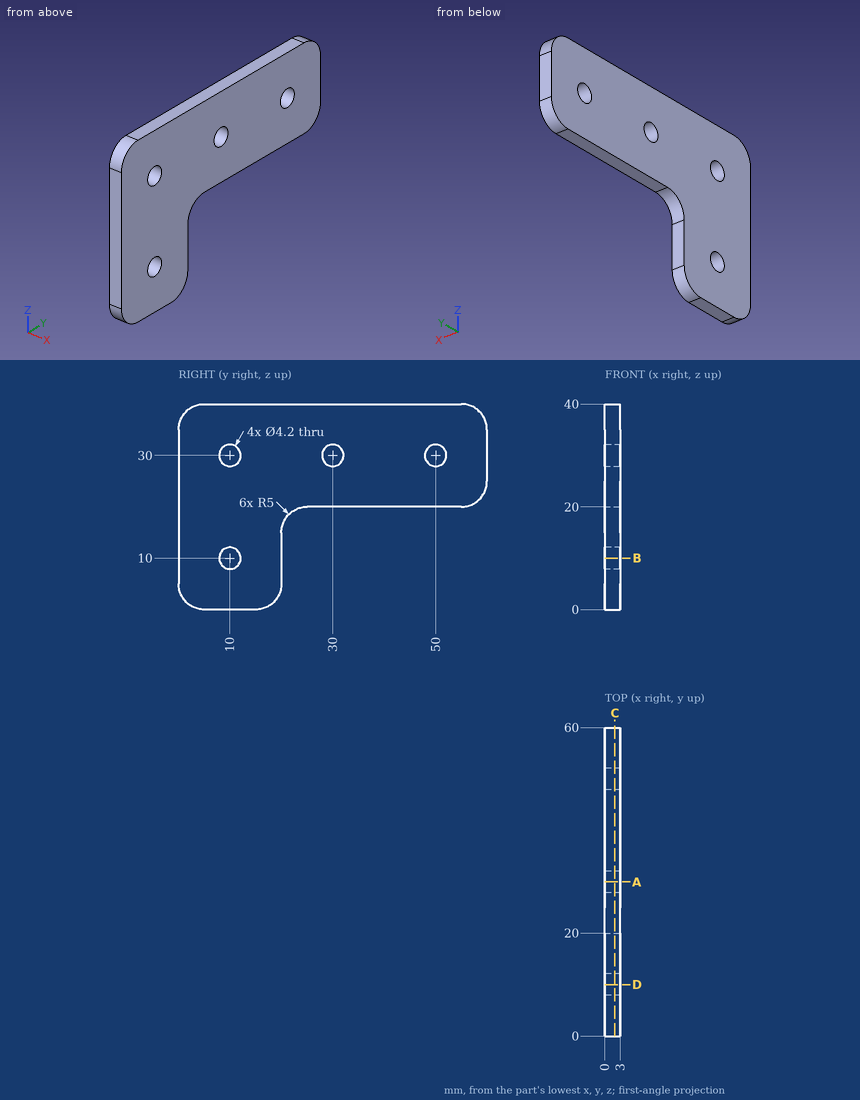
Source: three-view drawing plus pictorial views. Frame: mm from the lowest corner of the part. Give positions to 0.01 mm unless a question says otherwise; leave off trailing zeros. Order: outer loops, then holes, each group sorted by start corner. A loop starts at its lowest first (then second) coordinate and runs counter-clockwise, first axis right, second up. Notation, with made-up numbers: M 65.25,46.25 L 90.25,46.25 A26 ccw 90.25,73.25 Z; hole C 8.5,1 d4. An arc over 180 degrees is marked long. Return JSON: item names as keys, results as strings.
1) Section query D-D on y = 10. Output: boundary loops of the cut face in (x, z).
Taken from the geometry:
{"outline": "M 0,0 L 3,0 L 3,7.9 L 0,7.9 Z; M 0,12.1 L 3,12.1 L 3,27.9 L 0,27.9 Z; M 0,32.1 L 3,32.1 L 3,40 L 0,40 Z"}
2) Line query: L1, parallel to Y at x = 2.2, z = 30; L2, parallel to Z at x = 0.3, y = 54; L3, parallel to Z at x = 2.55, y = 11.5. Output: solid intervals per line, ascending. Write a range as [from, to].
Taken from the geometry:
{"L1": "y = [0, 7.9], [12.1, 27.9], [32.1, 47.9], [52.1, 60]", "L2": "z = [20, 40]", "L3": "z = [0, 8.53], [11.47, 28.53], [31.47, 40]"}
3) Section query B-B on z = 10. Output: boundary loops of the cut face in (x, y), and give its area (3 significant figures).
Taken from the geometry:
{"outline": "M 0,0 L 3,0 L 3,7.9 L 0,7.9 Z; M 0,12.1 L 3,12.1 L 3,20 L 0,20 Z", "area": "47.4 mm2"}
4) Section query C-C on x = 1.9. Output: boundary loops of the cut face in (y, z).
Taken from the geometry:
{"outline": "M 0,5 A5 ccw 5,0 L 15,0 A5 ccw 20,5 L 20,15 A5 cw 25,20 L 55,20 A5 ccw 60,25 L 60,35 A5 ccw 55,40 L 5,40 A5 ccw 0,35 Z; hole C 10,10 d4.2; hole C 10,30 d4.2; hole C 30,30 d4.2; hole C 50,30 d4.2"}
5) Section query A-A on y = 30. Output: boundary loops of the cut face in (x, z).
Taken from the geometry:
{"outline": "M 0,20 L 3,20 L 3,27.9 L 0,27.9 Z; M 0,32.1 L 3,32.1 L 3,40 L 0,40 Z"}
